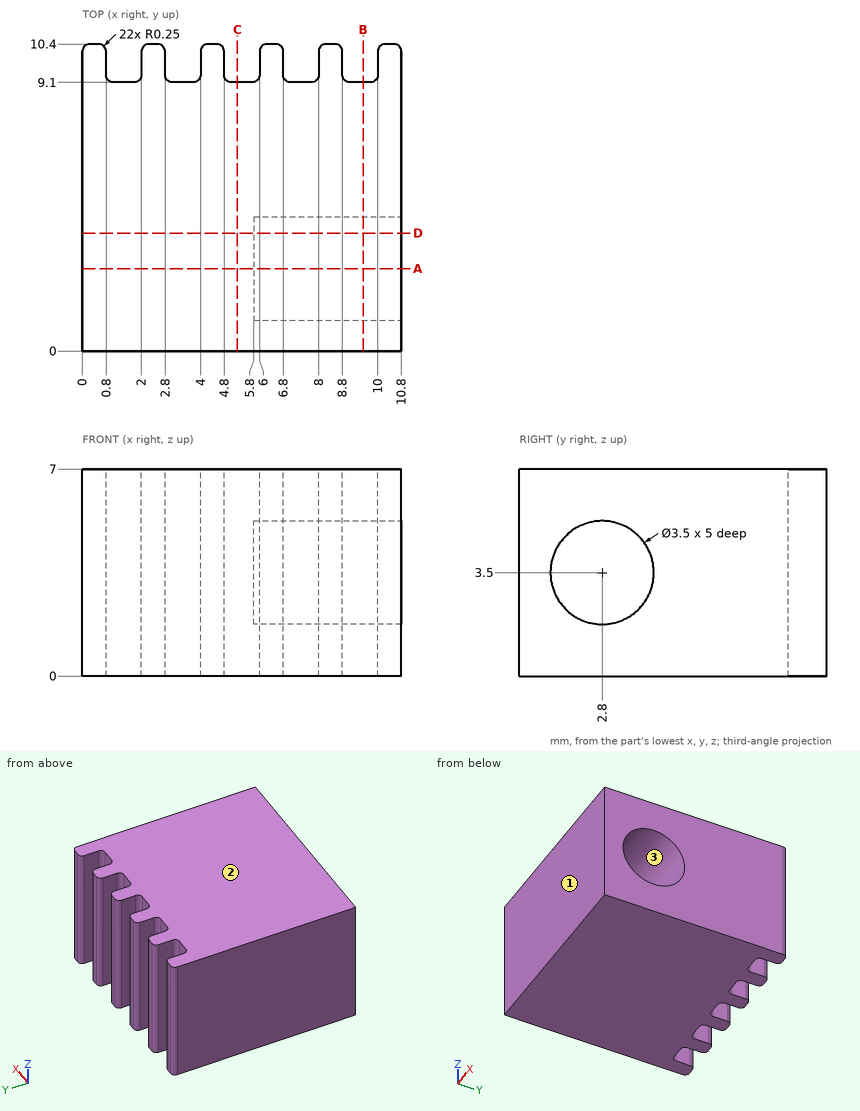
Geometry: see drawing. Coordinates: mm, zero at the bounding-box minimum. Round coordinates to 2 decimals unless told otherwise and drop trailing zeros. Order: outer loops, then holes, each group sorted by start corner. A loop starts at its lowest first (then second) coordinate and runs counter-clockwise, first axis right, second up. Notation, with made-up numbers: (-27.75, 39) - (-21.75, 39) arc R14 ccw to (-21.75, 63) - close; hole circle Ø6 at (-28.5, -14). An arc over 180 degrees is marked (long way). One line per question, with ' | ' between items. Start each with the question number.
1) Ray query, probe 1 along X at (y, z) = (1.5, 4); probe 2 along Y at (x, z) = (5.5, 5.5); probe 3 along Y at (x, z) = (8.25, 3.5). Return the intervals inside material, ascending.
2) Pull-direction query (Y, two-part tool) for the marked faces 1, 2 and 3; classes: +Y half, -Y half, draft (parallel to the pull), parting line (faces both ways), or undercut.
3) Cut plane B-B, the plane x = 9.5. Return the cut outline in (y, z).
4) Cut plane A-A, the plane y = 2.8. Return the cut outline in (x, z), then the cut area to 3 significant figures.
5) Cut plane D-D, the plane y = 4. Return the cut outline in (x, z).
6) Cut plane C-C, the plane x = 5.25. Return the cut outline in (y, z).
Worked out:
1) probe 1: x = 0 to 5.8 | probe 2: y = 0 to 9.1 | probe 3: y = 0 to 1.05, 4.55 to 10.4
2) face 1: -Y half | face 2: draft | face 3: undercut
3) outline: (0, 0) - (9.1, 0) - (9.1, 7) - (0, 7) - close; hole circle Ø3.5 at (2.8, 3.5)
4) outline: (0, 0) - (10.8, 0) - (10.8, 1.75) - (5.8, 1.75) - (5.8, 5.25) - (10.8, 5.25) - (10.8, 7) - (0, 7) - close | area: 58.1 mm^2
5) outline: (0, 0) - (10.8, 0) - (10.8, 2.23) - (5.8, 2.23) - (5.8, 4.77) - (10.8, 4.77) - (10.8, 7) - (0, 7) - close
6) outline: (0, 0) - (9.1, 0) - (9.1, 7) - (0, 7) - close
